from build123d import *

# Parameters (mm, degrees)
F0_W      = 30
F0_H      = 25
F1_DEPTH  = 17
F3_DEPTH  = 11
F4_R      = 3.75
F5_DEPTH  = 25
F6_W      = 8.5
F6_H      = 25
F7_DEPTH  = 12
F9_DEPTH  = 12
F10_R     = 1.8
F11_DEPTH = 8.5
F12_R     = 1.8
F13_DEPTH = 2.6
F15_DEPTH = 8
F16_R     = 1.8
F17_DEPTH = 14
F18_R     = 1.8
F19_DEPTH = 2.5
F21_SIZE  = 0.5
F22_SIZE2 = 1
F22_SIZE  = 1
F23_R     = 1.35
F24_DEPTH = 5.0024289632


# Not quite as in the source:
# - a feature names something its author has since deleted; it is built from what else it names


with BuildPart() as f1:
    # F0 (on Top) → F1 (new body)
    with BuildSketch(Plane.XY):
        Rectangle(F0_W, F0_H)
    extrude(amount=F1_DEPTH)

    # F2 (on face) → F3 (cut)
    with BuildSketch(Plane.XZ.offset(12.5)):
        Polygon((10, 17), (2, 17), (2, 3.5), (12, 3.5), (12, 11.5), (10, 13.5), align=None)
    extrude(amount=-F3_DEPTH, mode=Mode.SUBTRACT)

    # F4 (on face) → F5 (cut, through all)
    with BuildSketch(Plane.XZ.offset(12.5)):
        with Locations((-6.5, 8.5)):
            Circle(F4_R)
    extrude(amount=-F5_DEPTH, mode=Mode.SUBTRACT)

    # F6 (on face) → F7 (join)
    with BuildSketch(Plane.XY.offset(17)):
        with Locations((-10.75, 0)):
            Rectangle(F6_W, F6_H)
    extrude(amount=F7_DEPTH)

    # F8 (on face) → F9 (cut)
    with BuildSketch(Plane.XY.offset(29)):
        with BuildLine():
            Line((-6.5, -4.1892720131), (-6.5, 4.1892720131))
            ThreePointArc((-6.5, 4.1892720131), (-10.4, 0), (-6.5, -4.1892720131))
        make_face()
    extrude(amount=-F9_DEPTH, mode=Mode.SUBTRACT)

    # F10 (on face) → F11 (cut, through all)
    with BuildSketch(Plane.YZ.offset(-6.5)):
        with Locations((-8.3446360066, 23)):
            Circle(F10_R)
        with Locations((8.3446360066, 23)):
            Circle(F10_R)
    extrude(amount=-F11_DEPTH, mode=Mode.SUBTRACT)

    # F12 (on face) → F13 (cut)
    with BuildSketch(Plane(origin=(-15, 0, 0), x_dir=(0, -1, 0), z_dir=(-1, 0, 0))):
        Polygon((11.3446360067, 21.2679491924), (11.3446360067, 24.7320508076), (8.3446360067, 26.4641016151), (5.3446360067, 24.7320508076), (5.3446360067, 21.2679491924), (8.3446360067, 19.5358983849), align=None)
        with Locations((8.3446360066, 23)):
            Circle(F12_R, mode=Mode.SUBTRACT)
        Polygon((-5.3446360064, 21.2679491924), (-5.3446360064, 24.7320508076), (-8.3446360064, 26.4641016151), (-11.3446360064, 24.7320508076), (-11.3446360064, 21.2679491924), (-8.3446360064, 19.5358983849), align=None)
        with Locations((-8.3446360066, 23)):
            Circle(F12_R, mode=Mode.SUBTRACT)
    extrude(amount=-F13_DEPTH, mode=Mode.SUBTRACT)

    # F14 (on face) → F15 (cut)
    with BuildSketch(Plane.XY.offset(17)):
        with BuildLine():
            Line((5.95, 12.5), (4.5, 12.5))
            Line((4.5, 12.5), (4.5, 3.5))
            Line((4.5, 3.5), (5.95, 3.5))
            Line((5.95, 3.5), (5.95, 4.9))
            ThreePointArc((5.95, 4.9), (5.35, 5.5), (5.95, 6.1))
            Line((5.95, 6.1), (5.95, 6.9))
            ThreePointArc((5.95, 6.9), (5.35, 7.5), (5.95, 8.1))
            Line((5.95, 8.1), (5.95, 8.9))
            ThreePointArc((5.95, 8.9), (5.35, 9.5), (5.95, 10.1))
            Line((5.95, 10.1), (5.95, 10.9))
            ThreePointArc((5.95, 10.9), (5.35, 11.5), (5.95, 12.1))
            Line((5.95, 12.1), (5.95, 12.5))
        make_face()
    extrude(amount=-F15_DEPTH, mode=Mode.SUBTRACT)

    # F16 (on face) → F17 (cut, through all)
    with BuildSketch(Plane(origin=(0, 12.5, 0), x_dir=(-1, 0, 0), z_dir=(0, 1, 0))):
        with Locations((-9.3, 6.5)):
            Circle(F16_R)
    extrude(amount=-F17_DEPTH, mode=Mode.SUBTRACT)

    # F18 (on face) → F19 (cut)
    with BuildSketch(Plane(origin=(0, 12.5, 0), x_dir=(-1, 0, 0), z_dir=(0, 1, 0))):
        Polygon((-7.6256842194, 9.4), (-10.9743157806, 9.4), (-12.6486315613, 6.5), (-10.9743157806, 3.6), (-7.6256842194, 3.6), (-5.9513684387, 6.5), align=None)
        with Locations((-9.3, 6.5)):
            Circle(F18_R, mode=Mode.SUBTRACT)
    extrude(amount=-F19_DEPTH, mode=Mode.SUBTRACT)

    # F21
    f21_edges = [f1.edges().sort_by_distance(p)[0] for p in [
        (0, -12.5, 0),
        (-15, 0, 0),
        (0, 12.5, 0),
        (15, 0, 0),
        (-1, 12.5, 17),
        (10.475, 12.5, 17),
        (-15, 12.5, 14.5),
        (-15, -12.5, 14.5),
        (2, -12.5, 10.25),
        (-6.5, -12.5, 23),
        (7, -12.5, 3.5),
        (12, -12.5, 7.5),
        (11, -12.5, 12.5),
        (10, -12.5, 15.25),
        (15, -12.5, 8.5),
        (12.5, -12.5, 17),
        (15, 0, 17),
        (15, 12.5, 8.5),
        (-6.5, 12.5, 23),
        (-10.75, 12.5, 29),
        (-6.5, 8.344636, 29),
        (-6.5, -8.344636, 29),
        (-10.75, -12.5, 29),
        (-2.25, -12.5, 17),
        (-15, 0, 29),
        (-10.4, 0, 29),
    ]]
    chamfer(f21_edges, length=F21_SIZE)

    # F22
    f22_edges = [f1.edges().sort_by_distance(p)[0] for p in [
        (-2.75, 0, 8.5),
        (-10.25, -12.5, 8.5),
        (-10.25, 12.5, 8.5),
    ]]
    chamfer(f22_edges, length=F22_SIZE, length2=F22_SIZE2)

    # F23 (on face) → F24 (cut, through all)
    with BuildSketch(Plane(origin=(0, 0, 0), x_dir=(1, 0, 0), z_dir=(0, 0, -1))):
        with Locations((-6.5, 0)):
            Circle(F23_R)
    extrude(amount=-F24_DEPTH, mode=Mode.SUBTRACT)


solid = f1.part
The listing builds one solid part. Answer for the finished solid, in the listing's coordinates (mm). A direction names the side the tool comes from. Coordinates: 2 decimals unless noted, no trailing zeros. Order: outer loops, then holes, each group sorted by start corner. A loop starts at its lowest first (then second) coordinate and runs counter-clockwise, first axis right, second up.
Q1. Given P1, Ø11, axis at x = 7, y = -7, coming from the +Z side; P2, Ø6, axis at y = -8.5, z = 25, coming from the +X side; P3, Ø3, axis at y = -9.5, z = 22, coming from the -X side, each flat-ended and moving along its own axis, determine where each tip first touches the part or whether it passes through.
Q2. A cutting plane is placed at B-B, the plane z = 23. Write down the section's boundary in (x, y), and give its area (3 significant figures).
Q3. A cutting plane is placed at A-A, the plane y = 0. Write down the section's boundary in (x, z).
Q4. A cutting plane is placed at D-D, the plane y = -7.75. Write down the section's boundary in (x, z), and give its area (3 significant figures).
Q5. A cutting plane is placed at C-C, the plane y = 9.5. Write down the section's boundary in (x, z).
Q6. Which of the six approach directions +Z, -Z, +X, -X, +Y, -Y give full straight-line access (tool end or side, diameter ignored) to faces 1 (the face through (11.26, -12.25, 12.59)), 2 (the face through (-13.718, 6.866, 20.39)), 3 (the face through (10, -7, 15)), 4 (the face through (9, 11, 9.4))?
Q7. Consider line 1 (X direction, y = 0, z = 1.5); line 2 (Y direction, x = 5.5, z = 12.5); line 3 (Y direction, x = -7, z = 24.5). Determine where each line is inside the solid, lowest interval first.
Q8. For a pull along X with two mould halves and no side action, classify faces 5 (the face through (-14, 11.345, 23)), 6 (the face through (-15, 0, 14)), 7 (the face through (4.5, 8, 13)) as pulls with the +X half, pulls with the -X half, needs draft (parallel to the pull), parting line crosses it, or undercut.
Answers follow:
1. P1: stops at z = 17
1. P2: stops at x = -6.5
1. P3: stops at x = -12.4
2. outline: (-15, -12) - (-14.5, -12.5) - (-7, -12.5) - (-6.5, -12) - (-6.5, -10.14) - (-12.4, -10.14) - (-12.4, -11.34) - (-15, -11.34) - close; (-15, -5.34) - (-12.4, -5.34) - (-12.4, -6.54) - (-6.5, -6.54) - (-6.5, -4.19) arc R4.2 cw to (-6.5, 4.19) - (-6.5, 6.54) - (-12.4, 6.54) - (-12.4, 5.34) - (-15, 5.34) - close; (-15, 11.34) - (-12.4, 11.34) - (-12.4, 10.14) - (-6.5, 10.14) - (-6.5, 12) - (-7, 12.5) - (-14.5, 12.5) - (-15, 12) - close
2. area: 113 mm2
3. outline: (-15, 0.5) - (-14.5, 0) - (-7.85, 0) - (-7.85, 5) arc R3.75 cw (long way) to (-5.15, 5) - (-5.15, 0) - (14.5, 0) - (15, 0.5) - (15, 16.5) - (14.5, 17) - (-10.4, 17) - (-10.4, 28.5) - (-10.9, 29) - (-14.5, 29) - (-15, 28.5) - close; hole circle Ø3.6 at (9.3, 6.5)
4. outline: (-15, 0.5) - (-14.5, 0) - (14.5, 0) - (15, 0.5) - (15, 16.5) - (14.5, 17) - (10, 17) - (10, 13.5) - (12, 11.5) - (12, 3.5) - (2, 3.5) - (2, 17) - (-6.5, 17) - (-6.5, 21.3) - (-12.4, 21.3) - (-12.4, 19.88) - (-15, 19.88) - close; (-15, 26.12) - (-12.4, 26.12) - (-12.4, 24.7) - (-6.5, 24.7) - (-6.5, 28.5) - (-7, 29) - (-14.5, 29) - (-15, 28.5) - close; hole circle Ø7.5 at (-6.5, 8.5)
4. area: 405 mm2
5. outline: (-15, 0.5) - (-14.5, 0) - (14.5, 0) - (15, 0.5) - (15, 16.5) - (14.5, 17) - (5.35, 17) - (5.35, 9) - (4.5, 9) - (4.5, 17) - (-6.5, 17) - (-6.5, 21.62) - (-12.4, 21.62) - (-12.4, 20.2) - (-15, 20.2) - close; (-15, 25.8) - (-12.4, 25.8) - (-12.4, 24.38) - (-6.5, 24.38) - (-6.5, 28.5) - (-7, 29) - (-14.5, 29) - (-15, 28.5) - close; hole circle Ø7.5 at (-6.5, 8.5); hole circle Ø3.6 at (9.3, 6.5)
6. face 1: -Y
6. face 2: -X
6. face 3: +Z, -Y
6. face 4: +Y
7. line 1: x = -15 to -7.85, -5.15 to 15
7. line 2: y = -1.5 to 3.5, 5.1 to 5.9, 7.1 to 7.9, 9.1 to 9.9, 11.1 to 11.9
7. line 3: y = -12.5 to -9.34, -7.35 to -4.12, 4.12 to 7.35, 9.34 to 12.5
8. face 5: needs draft
8. face 6: pulls with the -X half
8. face 7: undercut
